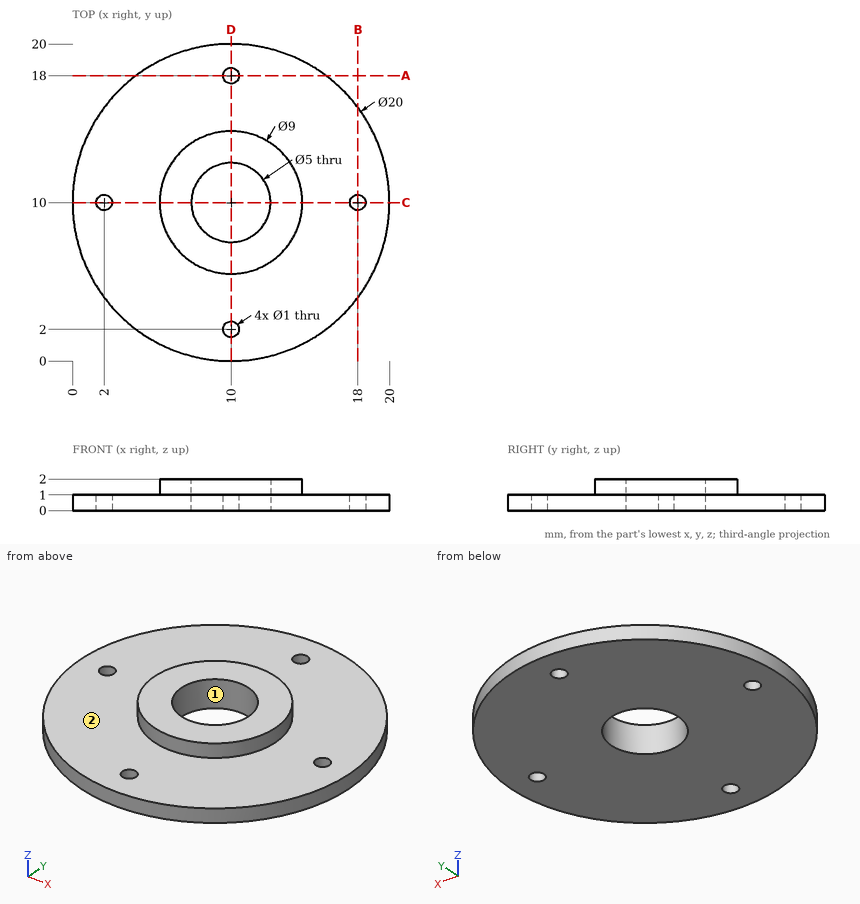
Job drawing, mm, ordinate dimensions from the low corner. One solid piece. Give positions to 0.01 mm unless a question says otherwise; leave off trailing zeros. Loops run counter-clockwise (first coordinate to the right, second up) from the corner with the lowest first, then second, coordinate; pieces in that order, holes last. Notation, with made-up numbers: (-21.5, 75) - (21.5, 75) arc R13 cw to (21.5, 89) - close; hole circle Ø4 at (-36.75, 78). An arc over 180 degrees is marked (long way). Use one line per item in the form item = value.
(1) Cut at A-A (y = 18). Give the cut face in (x, z).
Determined:
outline = (4, 0) - (9.5, 0) - (9.5, 1) - (4, 1) - close; (10.5, 0) - (16, 0) - (16, 1) - (10.5, 1) - close
(2) Drop flat-ended pins along their axis: P1, Ø2, axis at x = 7, y = 2.5, coming from the +Z side; P2, Ø1, axis at x = 13, z = 1, coming from the +Y side. Give the stop position or say it passes through.
Determined:
P1 = 1
P2 = 19.68
(3) Pull direction X, two halves, no side cores. Call the marked faces 1 and 2: pulls with the +X half, pulls with the -X half, needs draft (parallel to the pull), parting line crosses it, or undercut.
Determined:
face_1 = undercut
face_2 = needs draft
(4) Cut at C-C (y = 10). Give the cut face in (x, z).
Determined:
outline = (0, 0) - (1.5, 0) - (1.5, 1) - (0, 1) - close; (2.5, 0) - (7.5, 0) - (7.5, 2) - (5.5, 2) - (5.5, 1) - (2.5, 1) - close; (12.5, 0) - (17.5, 0) - (17.5, 1) - (14.5, 1) - (14.5, 2) - (12.5, 2) - close; (18.5, 0) - (20, 0) - (20, 1) - (18.5, 1) - close
(5) Drill centre lines: L1, parallel to Z at x = 17, y = 13; L2, parallel to Y at x = 18.25, z = 0.9; L3, parallel to Y at x = 11.5, z = 1.3. Where is each one in solid material? Low to high.
Determined:
L1 = 0 to 1
L2 = 4.35 to 9.57, 10.43 to 15.65
L3 = 5.76 to 8, 12 to 14.24
